Autodesk Inventor part; units mm, degrees
ref_plane "YZ Plane" through (0, 0, 0) normal (1, 0, 0) x (0, 1, 0)
ref_plane "XZ Plane" through (0, 0, 0) normal (0, 1, 0) x (-1, 0, 0)
ref_plane "XY Plane" through (0, 0, 0) normal (0, 0, 1) x (1, 0, 0)
sketch "Sketch3" plane through (0, 0, 0) normal (0, 1, 0) x (-1, 0, 0)
  line L0 (0, 0) -> (125, 0)
  line L1 (125, 0) -> (125, 125)
  line L2 (125, 125) -> (0, 125)
  line L3 (0, 125) -> (0, 0)
  dimension "d10" = 125
  dimension "d11" = 125
extrude "Extrusion3" add sketch "Sketch3" along normal blind 10
sketch "Sketch8" plane through (0, 10, 0) normal (0, 1, 0) x (1, 0, 0)
  line L0 (0, 0) -> (-125, 0)
  line L1 (0, 0) -> (-4, 0)
  line L2 (-4, 0) -> (-4, -121)
  line L3 (-125, -125) -> (0, -125)
  line L4 (-4, -121) -> (-125, -121)
  line L5 (-125, 0) -> (-125, -125)
  line L6 (0, 0) -> (-125, 0)
  line L7 (-125, 0) -> (-125, -125)
  line L8 (-125, -125) -> (0, -125)
  line L9 (0, -125) -> (0, 0)
  dimension "d38" = 4
  dimension "d39" = 121
  dimension "d40" = 90
extrude "Extrusion8" add sketch "Sketch8" along normal blind 125 contours L9 L3 L5 L4 L2 L0
sketch "Sketch9" plane through (-125, 0, 125) normal (0, 0, 1) x (1, 0, 0)
  line L0 (0, 0) -> (0, 10)
  line L1 (0, 10) -> (0, 30)
  line L2 (0, 0) -> (0, 135)
  line L3 (0, 30) -> (15, 30)
  line L4 (15, 30) -> (60, 30)
  line L5 (60, 30) -> (60, 52.5)
  line L6 (60, 52.5) -> (15, 52.5)
  line L7 (15, 52.5) -> (15, 30)
  line L8 (15, 52.5) -> (15, 62.5)
  line L9 (15, 62.5) -> (15, 85)
  line L10 (15, 85) -> (60, 85)
  line L11 (60, 85) -> (60, 62.5)
  line L12 (60, 62.5) -> (15, 62.5)
  line L13 (60, 62.5) -> (70, 62.5)
  line L14 (70, 62.5) -> (70, 85)
  line L15 (70, 85) -> (115, 85)
  line L16 (115, 85) -> (115, 62.5)
  line L17 (115, 62.5) -> (70, 62.5)
  line L18 (70, 52.5) -> (70, 62.5)
  line L19 (70, 52.5) -> (70, 30)
  line L20 (70, 30) -> (115, 30)
  line L21 (115, 30) -> (115, 52.5)
  line L22 (115, 52.5) -> (70, 52.5)
  point P0 (125, 0)
  dimension "d43" = 20
  dimension "d44" = 15
  dimension "d45" = 90
  dimension "d46" = 45
  dimension "d47" = 22.5
  dimension "d48" = 10
  dimension "d49" = 22.5
  dimension "d50" = 45
  dimension "d51" = 10
  dimension "d52" = 45
  dimension "d53" = 10
  dimension "d54" = 22.5
  dimension "d55" = 45
extrude "Extrusion9" cut sketch "Sketch9" against normal blind 10
sketch "Sketch10" plane through (-125, 0, 0) normal (-1, 0, 0) x (0, 0, 1)
  line L0 (0, 0) -> (125, 0)
  line L1 (125, 0) -> (125, 5)
  line L2 (0, 5) -> (0, 0)
  line L3 (125, 0) -> (125, 135)
  line L4 (125, 5) -> (10, 5)
  line L5 (10, 5) -> (10, 0)
  line L6 (0, 0) -> (125, 0)
  dimension "d59" = 5
  dimension "d62" = 125
  dimension "d63" = 115
extrude "Extrusion12" cut sketch "Sketch10" against normal blind 20
sketch "Sketch13" plane through (0, 10, 0) normal (0, 1, 0) x (1, 0, 0)
  line L0 (-125, -10) -> (-105, -10)
  line L1 (-125, -10) -> (-125, -47)
  line L2 (-4, -121) -> (-125, -121)
  line L3 (-125, -47) -> (-115, -47)
  line L4 (-115, -47) -> (-115, -84)
  point P0 (0, 0)
  dimension "d79" = 37
  dimension "d80" = 10
  dimension "d81" = 37
hole "Hole2" at (-115, 10, 84) at (-115, 10, 47) direction (0, -1, 0) diameter 4.318 end through all
sketch "Sketch14" plane through (0, 0, 0) normal (0, 0, -1) x (-1, 0, 0)
  line L0 (105, 0) -> (0, 0)
  line L1 (0, 0) -> (115, 0)
  line L2 (115, 0) -> (115, 5)
  line L3 (117.159, 5) -> (112.841, 5)
  line L4 (115, 5) -> (0, 5)
  line L5 (0, 0) -> (0, 135)
  line L6 (0, 0) -> (0, 5)
  dimension "d96" = 115
  dimension "d97" = 5
extrude "Extrusion14" add sketch "Sketch14" along normal blind 20
sketch "Sketch15" plane through (0, 10, 0) normal (0, 1, 0) x (1, 0, 0)
  line L0 (-115, 0) -> (-125, 0)
  line L1 (-115, 0) -> (-78, 0)
  line L2 (0, 0) -> (-115, 0)
  line L3 (-78, 0) -> (-78, 10)
  line L4 (-78, 10) -> (-41, 10)
  dimension "d100" = 37
  dimension "d101" = 10
  dimension "d102" = 37
hole "Hole3" at (-41, 10, -10) at (-78, 10, -10) direction (0, -1, 0) diameter 3.5 end through all
sketch "Sketch16" plane through (0, 0, 0) normal (0, -1, 0) x (1, 0, 0)
  line L0 (0, 0) -> (-115, 0)
  circle A0 centre (-41, -10) radius 1.75
  circle A1 centre (-78, -10) radius 1.75
  line L1 (-105, 10) -> (-125, 10)
  line L2 (-125, 0) -> (-125, 10)
  line L3 (-115, 0) -> (-125, 0)
  line L4 (-115, 0) -> (-115, -20)
  line L5 (0, -20) -> (-115, -20)
  line L6 (0, 125) -> (0, -20)
  line L7 (-105, 125) -> (0, 125)
  line L8 (-105, 125) -> (-105, 10)
extrude "Extrusion15" add sketch "Sketch16" along normal blind 3
sketch "Sketch17" plane through (0, -3, 0) normal (0, -1, 0) x (1, 0, 0)
  circle A0 centre (-41, -10) radius 1.75
  circle A1 centre (-78, -10) radius 1.75
  point P0 (0, 0)
hole "Hole4" at (-78, -3, -10) at (-41, -3, -10) direction (0, 1, 0) diameter 4.318 end through all counterbore diameter 7.62 counterbore depth 5.08
properties part number "QUarter1"
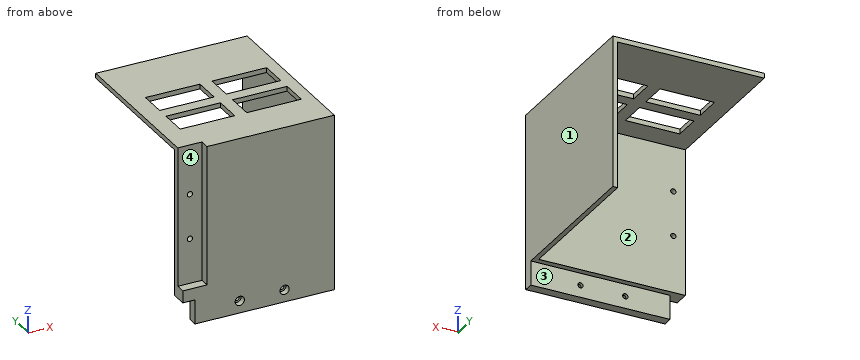
Check sheet for the modelled part. Datum: model origin and axes. Units: mm. Face numbers are marked on the shaded views. A direction names the side the tool comes from. Round coordinates to 2 decimals unless told otherwise and drop trailing zeros. Loops run counter-clockwise (first coordinate to the right, second up) from the corner with the lowest first, then second, coordinate; pieces in that order, holes last. Notation, with made-up numbers: (-30.75, 33) - (-26.75, 33) arc R32 ccw to (-26.75, 59) - close; hole circle Ø11 at (71, -9.75). An arc over 180 degrees is marked (long way). Write item = value, one per line. Start each with the question number.
Q1. Section check A-A (z = -10). Record the boundary of the cut face in (x, y).
Q2. Section check C-C (x = -28.5). Record the boundary of the cut face in (y, z), plus the area to 4 significant figures.
Q3. Section check B-B (y = 38.5). Record the boundary of the cut face in (x, z), plus the area to 3 significant figures.
Q4. Depth check by flat-ended pin: P1, Ø4, axis at x = -99.5, y = 14, coming from the -Z side; P2, Ø22, axis at x = -49, z = -9, coming from the +Y side; P3, Ø2.5, axis at x = -41, z = -10, coming from the +Y side; P4, Ø10, axis at x = -115.5, z = 86.5, coming from the -Y side. Enter the tip coordinate at first touch or a pass-through.
Q5. Thickness scan on L1, parallel to Z at x = -115, y = 7.9; L2, parallel to X at y = 3.3, z = -10; L3, parallel to X at y = -2, z = -10. Record the ranges inside material, lowest first.
Q6. Section check D-D (x = -78). Record the boundary of the cut face in (y, z), plus the area to 3 significant figures.
Q7. Access from +Z, -Z, +X, -X, +Y, -Y to the whole of each face (thin tool, end or side, straight path). Record for the marked faces 1, 2, 3 and 4.
Derived:
q1.outline = (-115, -3) - (-81.81, -3) - (-81.81, 2.08) - (-80.16, 2.08) - (-80.16, 5) - (-115, 5) - close; (-75.84, 2.08) - (-74.19, 2.08) - (-74.19, -3) - (-44.81, -3) - (-44.81, 2.08) - (-43.16, 2.08) - (-43.16, 5) - (-75.84, 5) - close; (-38.84, 2.08) - (-37.19, 2.08) - (-37.19, -3) - (0, -3) - (0, 5) - (-38.84, 5) - close
q2.outline = (-3, -20) - (5, -20) - (5, 0) - (10, 0) - (10, 121) - (30, 121) - (30, 125) - (-3, 125) - close; (52.5, 121) - (62.5, 121) - (62.5, 125) - (52.5, 125) - close; (85, 121) - (135, 121) - (135, 125) - (85, 125) - close
q2.area = 2,105 mm^2
q3.outline = (-125, 121) - (-110, 121) - (-110, 125) - (-125, 125) - close; (-65, 121) - (-55, 121) - (-55, 125) - (-65, 125) - close; (-10, 121) - (-4, 121) - (-4, 0) - (0, 0) - (0, 125) - (-10, 125) - close
q3.area = 624 mm^2
q4.P1 = 121
q4.P2 = 10
q4.P3 = through
q4.P4 = 5
q5.L1 = 0 to 44.84, 49.16 to 81.84, 86.16 to 125
q5.L2 = -115 to -80.16, -75.84 to -43.16, -38.84 to 0
q5.L3 = -115 to -81.81, -74.19 to -44.81, -37.19 to 0
q6.outline = (-3, -20) - (5, -20) - (5, -12.16) - (2.08, -12.16) - (2.08, -13.81) - (-3, -13.81) - close; (-3, -6.19) - (2.08, -6.19) - (2.08, -7.84) - (5, -7.84) - (5, 0) - (10, 0) - (10, 121) - (30, 121) - (30, 125) - (-3, 125) - close; (52.5, 121) - (62.5, 121) - (62.5, 125) - (52.5, 125) - close; (85, 121) - (135, 121) - (135, 125) - (85, 125) - close
q6.area = 2,050 mm^2
q7.face_1 = +Z, -Z, +X, +Y, -Y
q7.face_2 = -Z, -X, +Y
q7.face_3 = -Z, +X, -X, +Y
q7.face_4 = +Z, -X, -Y
